from build123d import *

# Parameters (mm, degrees)
F0_W          = 50.8
F0_H          = 127
F1_DEPTH      = 19.05
F2_W          = 50.8
F2_H          = 19.05
F3_DEPTH      = 6.35
F4_W          = 50.8
F4_H          = 19.05
F5_DEPTH      = 50.8
F7_DEPTH      = 19.051
F7_DEPTH_BACK = 107.951


with BuildPart() as f1:
    # F0 (on Top) → F1 (new body)
    with BuildSketch(Plane.XY):
        Rectangle(F0_W, F0_H)
    extrude(amount=F1_DEPTH)

    # F2 (on face) → F3 (cut)
    with BuildSketch(Plane.XY.offset(19.05)):
        with Locations((0, -47.625)):
            Rectangle(F2_W, F2_H)
    extrude(amount=-F3_DEPTH, mode=Mode.SUBTRACT)

    # F4 (on face) → F5 (join)
    with BuildSketch(Plane.XY.offset(19.05)):
        with Locations((0, 53.975)):
            Rectangle(F4_W, F4_H)
    extrude(amount=F5_DEPTH)

    # F6 (on face) → F7 (cut, two sides)
    with BuildSketch(Plane.XZ.offset(-44.45)) as f7_sk:
        Polygon((25.4, 69.85), (0, 69.85), (0, 50.8), align=None)
        Polygon((0, 50.8), (0, 69.85), (-25.4, 69.85), align=None)
    extrude(amount=-F7_DEPTH, mode=Mode.SUBTRACT)
    extrude(f7_sk.sketch, amount=-F7_DEPTH_BACK, mode=Mode.SUBTRACT)


solid = f1.part
Geometry check sheet. Reference: the model listing, model coordinates, mm. A direction names the side the tool comes from. Round coordinates to 2 decimals unless told otherwise and drop trailing zeros. Write each loop counter-clockwise with the first axis right and the second up, starting at its lowest first coordinate (ties: lowest second). Pieces come first, ordered by that corner, then holes. Notation, with made-up numbers: (50, 82.25) - (94, 82.25) arc R26 cw to (94, 120.25) - close; hole circle Ø8 at (85.5, -33). An arc over 180 degrees is marked (long way). One line per item, written item: value.
1. Cross-section at C-C on y = 53. Record the boundary of the cut face in (x, z).
The answers:
outline: (-25.4, 0) - (25.4, 0) - (25.4, 69.85) - (0, 50.8) - (-25.4, 69.85) - close
2. Cross-section at B-B on x = 21.5. Record the boundary of the cut face in (y, z) (3 decimals), and give its area (3 significant figures).
The answers:
outline: (-63.5, 0) - (63.5, 0) - (63.5, 66.925) - (44.45, 66.925) - (44.45, 19.05) - (-38.1, 19.05) - (-38.1, 12.7) - (-57.15, 12.7) - (-57.15, 19.05) - (-63.5, 19.05) - close
area: 3,210 mm^2
3. Cross-section at D-D on z = 22. Record the boundary of the cut face in (x, y), and give its area (3 significant figures).
The answers:
outline: (-25.4, 44.45) - (25.4, 44.45) - (25.4, 63.5) - (-25.4, 63.5) - close
area: 968 mm^2
4. Scan lines: L1, parallel to Y at x = -18, z = 16; L2, parallel to Y at x = -2.5, z = 50. Record each from-to range of solid material in increasing order.
The answers:
L1: y = -63.5 to -57.15, -38.1 to 63.5
L2: y = 44.45 to 63.5
5. Set-up check for faces 4 (the face through (0, 1, 0)), 5 (the face through (0, -38.1, 16)), 6 (the face through (0, -60, 19.05)), 7 (the face through (25.4, 13.2, 18.9)), 8 (the face through (12.52, 53.84, 60.19)): record each of +Z, -Z, +X, -X, +Y, -Y from which the full face is reachable in a straight line by a thin tool's end or side.
The answers:
face 4: -Z, +X, -X, +Y, -Y
face 5: +Z, +X, -X
face 6: +Z, +X, -X, -Y
face 7: +Z, -Z, +X, +Y, -Y
face 8: +Z, +Y, -Y
6. Mould release check, pull along X, two halves, no side actions. Record for faces 1 (the face through (0, -57.15, 16)), 2 (the face through (-12.88, 53.84, 60.46)), 3 (the face through (-25.4, 13.2, 18.9)): released by +X, released by -X, zero draft, split by the parting line, or undercut.
The answers:
face 1: zero draft
face 2: undercut
face 3: released by -X
7. Depth check by flat-ended pin: pin 1 Ø8 at (x, y) = (20, 40) entering from +Z; pin 2 Ø15 at (x, z) = (-12.5, 40) entering from -Y. Enter the tip coordinate at first touch or a pass-through.
The answers:
pin 1: stops at z = 19.05
pin 2: stops at y = 44.45
8. Cross-section at A-A on z = 59.5. Record the boundary of the cut face in (x, y).
The answers:
outline: (-25.4, 44.45) - (-11.6, 44.45) - (-11.6, 63.5) - (-25.4, 63.5) - close; (11.6, 44.45) - (25.4, 44.45) - (25.4, 63.5) - (11.6, 63.5) - close
